The drawing under review shows one solid part. Ordinate dimensions are in mm from its lowest x, y, z. Give positions to 0.01 mm unless a question says otherwise; leave off trailing zeros. Write each loop counter-clockwise with the first axis right and the second up, starting at its lowest first coordinate (ties: lowest second). Pieces come first, ordered by that corner, then holes. Notation, with made-up numbers: (57.5, -38.5) -> (90.5, -38.5) arc R18 ccw to (90.5, -22.5) -> close; hole circle Ø10 at (-5.75, 60). An arc over 180 degrees is marked (long way). Write item = value, one per line.
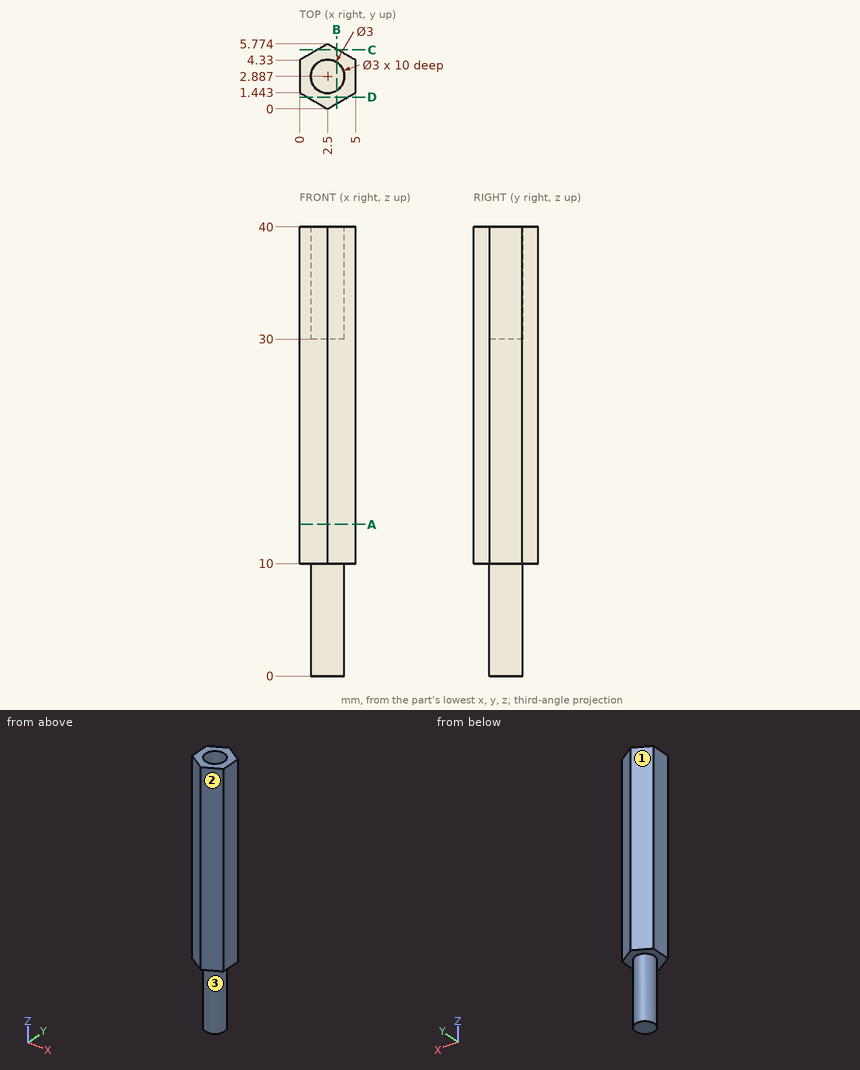
(1) The part is to be moulded in two halves that separate along X. For the marked faces 1, 2 and 3, say which applies: released by +X, released by -X, zero draft, split by the parting line, or undercut.
Answers below:
face_1 = released by -X
face_2 = released by +X
face_3 = split by the parting line
(2) Take a section at D-D (y = 1.05). Write out the cut boundary in (x, z).
Answers below:
outline = (0.68, 10) -> (4.32, 10) -> (4.32, 40) -> (0.68, 40) -> close
(3) Take a section at B-B (x = 3.3). Write out the cut boundary in (y, z) (1 decimal).
Answers below:
outline = (0.5, 10) -> (1.6, 10) -> (1.6, 0) -> (4.2, 0) -> (4.2, 10) -> (5.3, 10) -> (5.3, 40) -> (4.2, 40) -> (4.2, 30) -> (1.6, 30) -> (1.6, 40) -> (0.5, 40) -> close
(4) Take a section at C-C (y = 5.25). Write out the cut boundary in (x, z).
Answers below:
outline = (1.59, 10) -> (3.41, 10) -> (3.41, 40) -> (1.59, 40) -> close
(5) To check wall thickness, follow probe 1 along X at (y, z) = (2.8, 32.5); probe 2 along Z at (x, y) = (4.5, 2.95); probe 3 along Z at (x, y) = (2.45, 3.3). State the ranges of each line that lie inside material, in increasing order.
Answers below:
probe_1 = 0 to 1, 4 to 5
probe_2 = 10 to 40
probe_3 = 0 to 30
(6) Take a section at A-A (z = 13.5). Write out the cut boundary in (x, y).
Answers below:
outline = (0, 1.44) -> (2.5, 0) -> (5, 1.44) -> (5, 4.33) -> (2.5, 5.77) -> (0, 4.33) -> close
